For this review, use the dimensioned drawing (mm, ordinates from the lowest corner) and the shaded views. Coordinates: 2 decimals unless noted, no trailing zeros. Order: outer loops, then holes, each group sorted by start corner. A loop starts at its lowest first (then second) coordinate and runs counter-clockwise, first axis right, second up. Notation, with made-up numbers: M 47,75.5 L 74,75.5 A5 ccw 74,81.5 Z; hole C 85,51.25 d8. An arc over 180 degrees is marked long. Answer in a Markdown table with one row per item.
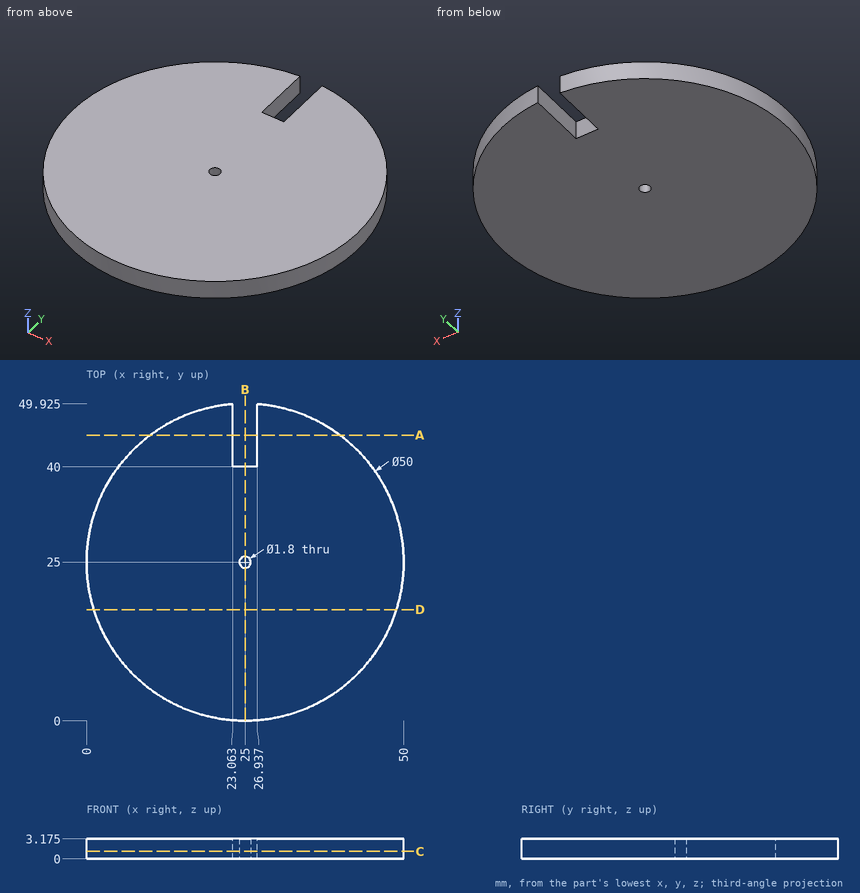
(1) Add section B-B, the plane x = 25. Give the boundary of the cut face in (y, z) (3 decimals).
Return value:
| item | result |
|---|---|
| outline | M 0,0 L 24.1,0 L 24.1,3.175 L 0,3.175 Z; M 25.9,0 L 40,0 L 40,3.175 L 25.9,3.175 Z |
(2) Insertion check: pin 1 Ø1.5 at (x, z) = (41.5, 1.5) entering from +Y (1 decimal); pin 2 Ø1 at (x, z) = (7.5, 2) entering from +Y; pin 3 Ø1.4 at (x, y) = (25, 25) entering from -Z; pin 4 Ø1 at (y, z) = (47, 1.5) entering from +X. Each pin has a flat end and moves straight along its axis. Give the tip position at first contact, or say it passes through.
Return value:
| item | result |
|---|---|
| pin 1 | stops at y = 44.4 |
| pin 2 | stops at y = 43.33 |
| pin 3 | passes through |
| pin 4 | stops at x = 37.76 |
(3) Add section D-D, the plane y = 17.5. Give the boundary of the cut face in (x, z) (1 decimal), and give its area (3 significant figures).
Return value:
| item | result |
|---|---|
| outline | M 1.2,0 L 48.8,0 L 48.8,3.2 L 1.2,3.2 Z |
| area | 151 mm2 |
(4) For line 1 along Y through (x, z) = (25, 1.15); line 2 along X through (y, z) = (46, 1) (1 decimal); line 3 along X through (y, z) = (47.5, 2.3), list the stretches that pass through material, from the lowest coordinate up. Write a range as from..to.
Return value:
| item | result |
|---|---|
| line 1 | y = 0..24.1, 25.9..40 |
| line 2 | x = 11.4..23.1, 26.9..38.6 |
| line 3 | x = 14.1..23.06, 26.94..35.9 |
(5) Add section C-C, the plane z = 1.2. Give the boundary of the cut face in (x, y) (3 decimals).
Return value:
| item | result |
|---|---|
| outline | M 23.063,40 L 23.063,49.925 A25 ccw long 26.937,49.925 L 26.937,40 Z; hole C 25,25 d1.8 |
(6) Add section A-A, the plane y = 45. Give the boundary of the cut face in (x, z) (3 decimals).
Return value:
| item | result |
|---|---|
| outline | M 10,0 L 23.063,0 L 23.063,3.175 L 10,3.175 Z; M 26.937,0 L 40,0 L 40,3.175 L 26.937,3.175 Z |
